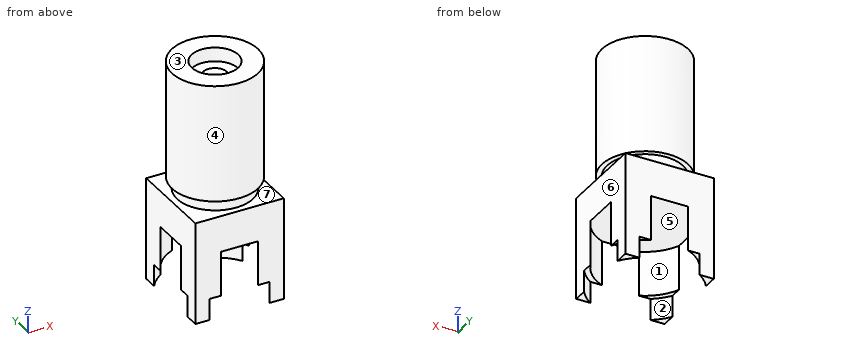
from build123d import *

# Parameters (mm, degrees)
SKETCH_W        = 9.5
SKETCH_H        = 9.5
PAD_DEPTH       = 11
SKETCH001_R     = 4.075
PAD001_DEPTH    = 1.3
SKETCH002_R     = 4.625
PAD002_DEPTH    = 12.6
SKETCH003_R     = 2.5
POCKET_DEPTH    = 1.5
SKETCH004_R     = 0.75
POCKET001_DEPTH = 5
SKETCH005_R     = 5.75
POCKET002_DEPTH = 2.3
SKETCH006_R     = 5.15
POCKET003_DEPTH = 4.8
CHAMFER_SIZE    = 0.5


with BuildPart() as part:
    # Sketch → Pad (new body)
    with BuildSketch(Plane.XY):
        Rectangle(SKETCH_W, SKETCH_H)
    extrude(amount=-PAD_DEPTH)

    # Sketch001 (on Face5 of Pad) → Pad001 (join)
    with BuildSketch(Plane.XY):
        Circle(SKETCH001_R)
    extrude(amount=PAD001_DEPTH)

    # Sketch002 (on Face8 of Pad001) → Pad002 (join)
    with BuildSketch(Plane.XY.offset(1.3)):
        Circle(SKETCH002_R)
    extrude(amount=PAD002_DEPTH)

    # Sketch003 (on Face3 of Pad002) → Pocket (cut)
    with BuildSketch(Plane.XY.offset(13.9)):
        Circle(SKETCH003_R)
    extrude(amount=-POCKET_DEPTH, mode=Mode.SUBTRACT)

    # Sketch004 (on Face7 of Pocket) → Pocket001 (cut)
    with BuildSketch(Plane.XY.offset(12.4)):
        Circle(SKETCH004_R)
    extrude(amount=-POCKET001_DEPTH, mode=Mode.SUBTRACT)

    # Sketch005 (on Face13 of Pocket001) → Pocket002 (cut)
    with BuildSketch(Plane(origin=(0, 0, -11), x_dir=(1, 0, 0), z_dir=(0, 0, -1))):
        Circle(SKETCH005_R)
    extrude(amount=-POCKET002_DEPTH, mode=Mode.SUBTRACT)

    # Sketch006 (on Face15 of Pocket002) → Pocket003 (cut)
    with BuildSketch(Plane(origin=(0, 0, -8.7), x_dir=(1, 0, 0), z_dir=(0, 0, -1))):
        Circle(SKETCH006_R)
    extrude(amount=-POCKET003_DEPTH, mode=Mode.SUBTRACT)

    # Chamfer
    chamfer_edges = [part.edges().sort_by_distance(p)[0] for p in [
        (-0.75, 0, 12.4),
    ]]
    chamfer(chamfer_edges, length=CHAMFER_SIZE)


solid = part.part
For this review, take the finished solid that the model builds, in its own axes (mm). Face numbers are marked on the shaded views. A direction names the side the tool comes from. Give positions to 0.01 mm unless a question says otherwise; leave off trailing zeros. Write each loop counter-clockwise with the first axis right and the second up, starting at its lowest first coordinate (ties: lowest second). Pieces come first, ordered by that corner, then holes. Notation, with made-up numbers: (40.25, 74) -> (94.25, 74) arc R9 ccw to (94.25, 87) -> close; hole circle Ø9 at (45, 72). An arc over 180 degrees is marked (long way). Use CSV: the item, a comma, the result in double quotes.
Q1. To check wall thickness, follow probe 1 along Y at (x, z) = (0, 8.8) (3 decimals); probe 2 along Y at (x, z) = (0, 13.1) (3 decimals); probe 3 along Z at (x, y) = (2.75, 0.5). State the ranges of each line that lie inside material, in increasing order. Write a range as [from, to].
Conclusion:
probe 1,"[-4.625, -0.75], [0.75, 4.625]"
probe 2,"[-4.625, -2.5], [2.5, 4.625]"
probe 3,"[-3.9, 13.9]"
Q2. For P1, Ø4.5, axis at x = 0, y = 0, coming from the -Z side; P2, Ø1.6, axis at x = 0, y = -0.5, coming from the +Z side; P3, Ø3, axis at x = -3.5, z = 7, coming from the +Y side, all flat-tipped, find the tip position at first contact; note any pin that passes through.
Conclusion:
P1,"z = -3.9"
P2,"z = 12.4"
P3,"y = 4.17"
Q3. Tool access review of the marked faces 5, 6 and 7: name each direction out of +Z, -Z, +X, -X, +Y, -Y from which nothing blocks a thin tool from reaching the whole face with its end or side.
Conclusion:
face 5,"-Z"
face 6,"+Z, -Z, +X, +Y, -Y"
face 7,"none"
Q4. Take a section at D-D, the plane z = 9.75. Write out the cut boundary in (x, y) (3 decimals), then the cut area to 3 significant figures.
Conclusion:
outline,"circle Ø9.25 at (0, 0); hole circle Ø1.5 at (0, 0)"
area,"65.4 mm2"
Q5. Take a section at A-A, the plane x = 0. Write out the cut boundary in (y, z) (3 decimals).
Conclusion:
outline,"(-4.75, -3.9) -> (4.75, -3.9) -> (4.75, 0) -> (4.075, 0) -> (4.075, 1.3) -> (4.625, 1.3) -> (4.625, 13.9) -> (2.5, 13.9) -> (2.5, 12.4) -> (1.25, 12.4) -> (0.75, 11.9) -> (0.75, 7.4) -> (-0.75, 7.4) -> (-0.75, 11.9) -> (-1.25, 12.4) -> (-2.5, 12.4) -> (-2.5, 13.9) -> (-4.625, 13.9) -> (-4.625, 1.3) -> (-4.075, 1.3) -> (-4.075, 0) -> (-4.75, 0) -> close"
Q6. Take a section at B-B, the plane z = -5.5. Write out the cut boundary in (x, y), then the cut area to 3 significant figures.
Conclusion:
outline,"(-4.75, -4.75) -> (-1.99, -4.75) arc R5.15 cw to (-4.75, -1.99) -> close; (-4.75, 1.99) arc R5.15 cw to (-1.99, 4.75) -> (-4.75, 4.75) -> close; (1.99, -4.75) -> (4.75, -4.75) -> (4.75, -1.99) arc R5.15 cw to start; (1.99, 4.75) arc R5.15 cw to (4.75, 1.99) -> (4.75, 4.75) -> close"
area,"11.2 mm2"
Q7. Mouldability with a two-part tool opening along X and no side actions: class the marked faces 1, 2, 3 and 4 as pulls with the +X half, pulls with the -X half, needs draft (parallel to the pull), parting line crosses it, or undercut.
Conclusion:
face 1,"undercut"
face 2,"undercut"
face 3,"needs draft"
face 4,"parting line crosses it"
